from build123d import *

# Parameters (mm, degrees)
SKETCH_1_R      = 2
SKETCH_1_R_2    = 2.5
SKETCH_1_R_3    = 1.5
SKETCH_1_R_4    = 4
EXTRUDE_1_DEPTH = 5
FILLET_1_R      = 2
FILLET_2_R      = 20


with BuildPart() as part:
    # 草图1 → 凸台-拉伸1 (new body)
    with BuildSketch(Plane.XY):
        Polygon((68.594555656, 79.826424772), (0, 108.239220029), (-76.536686473, 76.536686473), (-104.949481731, 7.942130817), (-81.001271248, 17.861804393), (-44.646345173, -69.906751195), (-68.594555656, -79.826424772), (0, -108.239220029), (76.536686473, -76.536686473), (104.949481731, -7.942130817), (81.001271248, -17.861804393), (44.646345173, 69.906751195), align=None)
        with Locations((-35.206875778, -84.996916991)):
            Circle(SKETCH_1_R, mode=Mode.SUBTRACT)
        with Locations((-25.113558797, -72.63992817)):
            Circle(SKETCH_1_R_2, mode=Mode.SUBTRACT)
        Polygon((-16.765813956, -71.888159542), (-18.679231118, -67.26876188), (-4.82103813, -61.528510394), (-2.907620968, -66.147908057), align=None, mode=Mode.SUBTRACT)
        with Locations((-60.249143904, -8.720129522)):
            Circle(SKETCH_1_R_3, mode=Mode.SUBTRACT)
        with Locations((-48.768640933, -36.436515497)):
            Circle(SKETCH_1_R_3, mode=Mode.SUBTRACT)
        with Locations((-2.008604821, -40.880502769)):
            Circle(SKETCH_1_R_4, mode=Mode.SUBTRACT)
        with Locations((-19.964230183, -38.035240412)):
            Circle(SKETCH_1_R_2, mode=Mode.SUBTRACT)
        with Locations((-26.595532152, -27.25211312)):
            Circle(SKETCH_1_R_3, mode=Mode.SUBTRACT)
        Polygon((-15.508977762, -22.659911932), (-26.989480733, 5.056474043), (-18.674564941, 8.500624935), (-7.19406197, -19.215761041), align=None, mode=Mode.SUBTRACT)
        with Locations((18.273617094, -89.846117992)):
            Circle(SKETCH_1_R_4, mode=Mode.SUBTRACT)
        with Locations((50.609400732, -76.45219786)):
            Circle(SKETCH_1_R_4, mode=Mode.SUBTRACT)
        with Locations((30.327178816, -27.486582637)):
            Circle(SKETCH_1_R_4, mode=Mode.SUBTRACT)
        Polygon((48.829632852, -44.717635844), (46.91621569, -40.098238182), (60.774408678, -34.357986696), (62.68782584, -38.977384359), align=None, mode=Mode.SUBTRACT)
        Polygon((-11.616485342, -37.283471784), (-13.529902504, -32.664074122), (32.664074122, -13.529902504), (34.577491284, -18.149300166), align=None, mode=Mode.SUBTRACT)
        with Locations((41.011818963, -12.778133876)):
            Circle(SKETCH_1_R_2, mode=Mode.SUBTRACT)
        with Locations((38.076035123, -0.464272855)):
            Circle(SKETCH_1_R_3, mode=Mode.SUBTRACT)
        with Locations((69.122153519, -33.606218069)):
            Circle(SKETCH_1_R_2, mode=Mode.SUBTRACT)
        with Locations((84.996916991, -35.206875778)):
            Circle(SKETCH_1_R, mode=Mode.SUBTRACT)
        with Locations((-84.996916991, 35.206875778)):
            Circle(SKETCH_1_R, mode=Mode.SUBTRACT)
        with Locations((-69.122153519, 33.606218069)):
            Circle(SKETCH_1_R_2, mode=Mode.SUBTRACT)
        with Locations((-38.076035123, 0.464272855)):
            Circle(SKETCH_1_R_3, mode=Mode.SUBTRACT)
        with Locations((-41.011818963, 12.778133876)):
            Circle(SKETCH_1_R_2, mode=Mode.SUBTRACT)
        Polygon((13.529902504, 32.664074122), (-32.664074122, 13.529902504), (-34.577491284, 18.149300166), (11.616485342, 37.283471784), align=None, mode=Mode.SUBTRACT)
        Polygon((-46.91621569, 40.098238182), (-60.774408678, 34.357986696), (-62.68782584, 38.977384359), (-48.829632852, 44.717635844), align=None, mode=Mode.SUBTRACT)
        with Locations((-30.327178816, 27.486582637)):
            Circle(SKETCH_1_R_4, mode=Mode.SUBTRACT)
        with Locations((-50.609400732, 76.45219786)):
            Circle(SKETCH_1_R_4, mode=Mode.SUBTRACT)
        with Locations((-18.273617094, 89.846117992)):
            Circle(SKETCH_1_R_4, mode=Mode.SUBTRACT)
        Polygon((18.674564941, -8.500624935), (7.19406197, 19.215761041), (15.508977762, 22.659911932), (26.989480733, -5.056474043), align=None, mode=Mode.SUBTRACT)
        with Locations((26.595532152, 27.25211312)):
            Circle(SKETCH_1_R_3, mode=Mode.SUBTRACT)
        with Locations((19.964230183, 38.035240412)):
            Circle(SKETCH_1_R_2, mode=Mode.SUBTRACT)
        with Locations((2.008604821, 40.880502769)):
            Circle(SKETCH_1_R_4, mode=Mode.SUBTRACT)
        with Locations((48.768640933, 36.436515497)):
            Circle(SKETCH_1_R_3, mode=Mode.SUBTRACT)
        with Locations((60.249143904, 8.720129522)):
            Circle(SKETCH_1_R_3, mode=Mode.SUBTRACT)
        Polygon((4.82103813, 61.528510394), (2.907620968, 66.147908057), (16.765813956, 71.888159542), (18.679231118, 67.26876188), align=None, mode=Mode.SUBTRACT)
        with Locations((25.113558797, 72.63992817)):
            Circle(SKETCH_1_R_2, mode=Mode.SUBTRACT)
        with Locations((35.206875778, 84.996916991)):
            Circle(SKETCH_1_R, mode=Mode.SUBTRACT)
    extrude(amount=EXTRUDE_1_DEPTH)

    # 圆角1
    fillet_1_edges = [part.edges().sort_by_distance(p)[0] for p in [
        (104.949481731, -7.942130817, 2.5),
        (-68.594555656, -79.826424772, 2.5),
        (-104.949481731, 7.942130817, 2.5),
        (68.594555656, 79.826424772, 2.5),
    ]]
    fillet(fillet_1_edges, radius=FILLET_1_R)

    # 圆角2
    fillet_2_edges = [part.edges().sort_by_distance(p)[0] for p in [
        (76.536686473, -76.536686473, 2.5),
        (0, -108.239220029, 2.5),
        (-76.536686473, 76.536686473, 2.5),
        (0, 108.239220029, 2.5),
    ]]
    fillet(fillet_2_edges, radius=FILLET_2_R)


solid = part.part
Could you check a few things on this model? Use its own coordinates, in mm. A direction names the side the tool comes from. Give positions to 0.01 mm unless a question says otherwise; leave off trailing zeros. Order: outer loops, then holes, each group sorted by start corner. A loop starts at its lowest first (then second) coordinate and runs counter-clockwise, first axis right, second up.
1. For faces 1 (the flat face through (11.293, 20.914, 2.465)), 2 (the flat face through (54.254, 73.886, 2.465)), which set-ups out of +Z, -Z, +X, -X, +Y, -Y let a thin tool reach every point of the face, with its end or its side?
2. Suppose I cut it at C-C (x = -76). List the corners of the cut face in (y, z) for me, plus the area to 3 significant figures.
3. Suppose I cut it at A-A (z = 2.5). Give the number of separate pieces and of enclosed holes in the cut face, plus the area to 3 significant figures.
4. Suppose I cut it at B-B (y = 51). List the corners of the cut face in (x, z) for me.
5. Will these pins go through, and if not, where does the flat tip stop? P1, Ø1, axis at y = 15.5, z = 2.5, coming from the -X side; P2, Ø1, axis at y = 70.5, z = 2, coming from the -X side; P3, Ø3, axis at x = 60, z = 2, coming from the +Y side.
6. We'd pull the mould along Y, two halves only. Please class faces 3 (the cylindrical face through (0.11, 106.59, 2.54)), 4 (the cylindrical face through (-43.51, 12.89, 2.46)), 5 (the flat face through (13, 5.2, 2.5)): pulls with the +Y half, pulls with the -Y half, needs draft (parallel to the pull), parting line crosses it, or undercut.
7. I need wall thicknesses on L1, parallel to Y at x = -52.5, z = 2.15; L2, parallel to Y at x = -5, z = 2.45; L3, parallel to X at y = -40, z = 2.85. Which ranges of each line are inside material? Lowest first, please.
Solved:
1. face 1: +Z, -Z
1. face 2: +Z, -Z, +X
2. outline: (5.79, 0) - (74.71, 0) - (74.71, 5) - (5.79, 5) - close
2. area: 345 mm2
3. separate pieces: 1
3. enclosed holes: 36
3. area: 25,100 mm2
4. outline: (-87.11, 0) - (52.48, 0) - (52.48, 5) - (-87.11, 5) - close
5. P1: stops at x = -102.03
5. P2: stops at x = -79.2
5. P3: stops at y = 84.01
6. face 3: pulls with the +Y half
6. face 4: undercut
6. face 5: undercut
7. L1: y = -86.49 to -73.16, -50.95 to 37.79, 43.2 to 72.93, 79.98 to 86.49
7. L2: y = -105.96 to -67.01, -61.6 to -43.54, -38.23 to -34.54, -29.13 to 24.99, 30.4 to 105.96
7. L3: x = -57.03 to -21.51, -18.42 to -5.91, 1.89 to 47.15, 60.22 to 91.67
